Could you check a few things on this model? Use its own coordinates, in mm. A direction names the side the tool comes from. Coordinates: 2 decimals unless noted, no trailing zeros. Write each loop counter-clockwise with the first axis right and the second up, starting at its lowest first coordinate (ties: lowest second). Pieces come first, ordered by that corner, then holes. Notation, with made-up numbers: M 14,85 L 37,85 A17 cw 37,108 Z; hole C 9,2.25 d11. An arc over 180 degrees is marked long. Answer as CSV lines item,"result". Start each with the question number.
Item 1: Suppose I cut it at A-A, the plane y = 0. Write out the boundary of the cut face in (x, z), and give its area (3 significant figures).
Item 2: Suppose I cut it at D-D, the plane z = 28.5. Write out the boundary of the cut face in (x, y).
Item 3: I'm going to push flat-ended pins straight in: P1, Ø7.5, axis at x = -5, y = -2.5, coming from the -Z side; P2, Ø8, axis at x = 17, z = 11, coming from the +Y side; P3, Ø10, axis at y = 15.5, z = 30, coming from the +X side. Where does each tip first touch, or does it pass through?
Item 4: We'd pull the mould along Y, two halves only. Please class faces 1 (the flat face through (0.1, -3.2, 20)), 2 (the cylindrical face through (10.382, -19.961, 20.14)), 3 (the flat face through (-12, -13, 10)): +Y half, -Y half, draft (parallel to the pull), parting line (faces both ways), or undercut.
Item 5: Suppose I cut it at C-C, the plane z = 16.5. Write out the boundary of the cut face in (x, y), and give its area (3 significant figures).
Item 6: If I drill on line 1 along Y through (x, z) = (0, 17); line 2 along Y through (x, z) = (0, 30); line 3 along Z through (x, y) = (17, 5.5), over which ranges is the centre line in solid material (lowest first)? Write a range as [from, to].
Item 7: On a 3-axis mill with a long thin cutter (end or side, diameter ignored), from which of +Z, -Z, +X, -X, +Y, -Y can I reach the whole of each face in a straight line? I mean faces 4 (the flat face through (0, -8, 35)), 5 (the cylindrical face through (-7.493, 0.33, 27.605)), 6 (the cylindrical face through (-13.887, -10.648, 5.07)). Say none if no direction works.
```python
from build123d import *

# Parameters (mm, degrees)
F0_W   = 4.5
F0_H   = 7
F0_W_2 = 5
F0_H_2 = 3
F0_H_3 = 15
F0_H_4 = 10
F2_R   = 5


with BuildPart() as f1:
    # F0 (on Front) → F1 (revolve)
    with BuildSketch(Plane.XZ):
        with Locations((5.25, 16.5)):
            Rectangle(F0_W, F0_H)
        with Locations((20, 11.5)):
            Rectangle(F0_W_2, F0_H_2)
        with Locations((20, 16.5)):
            Rectangle(F0_W_2, F0_H)
        with Locations((20, 27.5)):
            Rectangle(F0_W_2, F0_H_3)
        with Locations((15, 27.5)):
            Rectangle(F0_W_2, F0_H_3)
        with Locations((10, 27.5)):
            Rectangle(F0_W_2, F0_H_3)
        with Locations((10, 16.5)):
            Rectangle(F0_W_2, F0_H)
        with Locations((15, 16.5)):
            Rectangle(F0_W_2, F0_H)
        with Locations((15, 5)):
            Rectangle(F0_W_2, F0_H_4)
        with Locations((15, 11.5)):
            Rectangle(F0_W_2, F0_H_2)
    revolve(axis=Axis((0, 0, 17.5), (0, 0, 1)))

    # F2
    f2_edges = [f1.edges().sort_by_distance(p)[0] for p in [
        (-22.5, 0, 35),
    ]]
    fillet(f2_edges, radius=F2_R)


solid = f1.part
```
Ans:
1,outline,"M -22.5,10 L -17.5,10 L -17.5,0 L -12.5,0 L -12.5,13 L -3,13 L -3,20 L -7.5,20 L -7.5,35 L -17.5,35 A5 ccw -22.5,30 Z; M 3,13 L 12.5,13 L 12.5,0 L 17.5,0 L 17.5,10 L 22.5,10 L 22.5,30 A5 ccw 17.5,35 L 7.5,35 L 7.5,20 L 3,20 Z"
1,area,"872 mm^2"
2,outline,"C 0,0 d45; hole C 0,0 d15"
3,P1,"stops at z = 13"
3,P2,"stops at y = 18.36"
3,P3,"stops at x = 19.9"
4,face 1,"undercut"
4,face 2,"parting line"
4,face 3,"draft"
5,outline,"C 0,0 d45; hole C 0,0 d6"
5,area,"1,560 mm^2"
6,line 1,"y = [-22.5, -3], [3, 22.5]"
6,line 2,"y = [-22.5, -7.5], [7.5, 22.5]"
6,line 3,"z = [10, 34.99]"
7,face 4,"+Z, +X, -X, +Y, -Y"
7,face 5,"+Z"
7,face 6,"-Z"
